The listing builds one solid part. Answer for the finished solid, in the listing's coordinates (mm). Face numbers are marked on the shaded views. Coordinates: 2 decimals unless noted, no trailing zeros. Loops run counter-clockwise (first coordinate to the right, second up) from the corner with the lowest first, then second, coordinate; pieces in that order, holes last. Notation, with made-up numbers: (-19, -29.75) - (5, -29.75) arc R34 cw to (5, 4.25) - close; hole circle Ø3 at (-36, 81). An arc over 180 degrees is marked (long way). Write each question's results on one line, items separated by ' | '. Start each with the question number.
(1) Given pin 1 Ø10.5 at (y, z) = (16, -26) entering from -X; pin 2 Ø5 at (x, z) = (-0.5, 25.4) entering from +Y; pin 3 Ø8 at (y, z) = (23, 2) entering from +X; pin 4 Ø3.5 at (x, z) = (-0.5, -25.4) entering from -Y, each flat-ended and moving along its own axis, determine where each tip first touches the part or whether it passes through.
(2) Find section A-A on y = 21. Determine the outline of the cut face in (x, z), then the cut area to 3 significant figures.
(3) Determine the mould class of the marked faces 1, 2 and 3 for opening direction X: released by +X, released by -X, zero draft, split by the parting line, or undercut.
(4) Find section C-C on z = -6.5. Determine the outline of the cut face in (x, y), then the cut area to 3 significant figures.
(5) Find section D-D on x = -0.5. State how many separate pieces and enclosed holes the cut face has, then the cut area to 3 significant figures.
(6) Consider line 1 (X direction, y = 8, z = 25.4) (3 decimals); line 2 (X direction, y = 6, z = 0) (3 decimals); line 3 (Z direction, x = 13, y = 27). Determine where each line is inside the solid, lowest interval first. Write a range as from..to.
(7) Find section B-B on z = 25.4. Determine the outline of the cut face in (x, y) (3 decimals).
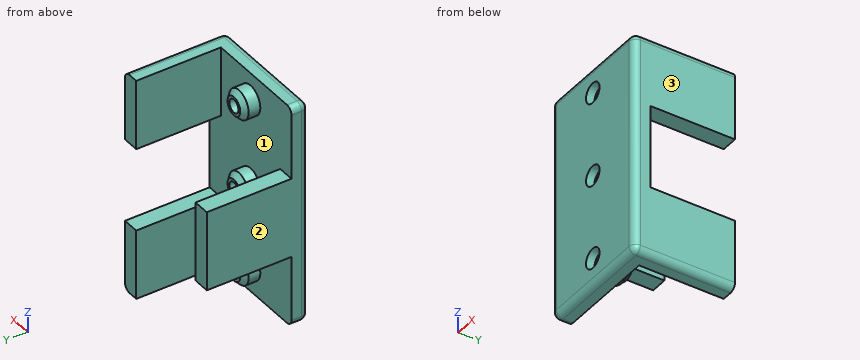
Autodesk Inventor part; units mm, degrees
ref_plane "YZ Plane" through (0, 0, 0) normal (1, 0, 0) x (0, 1, 0)
ref_plane "XZ Plane" through (0, 0, 0) normal (0, 1, 0) x (-1, 0, 0)
ref_plane "XY Plane" through (0, 0, 0) normal (0, 0, 1) x (1, 0, 0)
sketch "Sketch1" plane through (0, 0, 0) normal (0, 1, 0) x (-1, 0, 0)
  line L0 (18.7, 33.5) -> (-17.7, 33.5)
  line L1 (-17.7, 33.5) -> (-17.7, -33.5)
  line L2 (-17.7, -33.5) -> (18.7, -33.5)
  line L3 (18.7, -33.5) -> (18.7, 33.5)
  point P0 (0, 0)
  dimension "d0" = 36.4
  dimension "d1" = 67
extrude "Extrusion1" add sketch "Sketch1" along normal blind 5
sketch "Sketch2" plane through (0, 5, 0) normal (0, 1, 0) x (1, 0, 0)
  line L0 (-18.7, -33.5) -> (17.7, -33.5)
  line L1 (17.7, -33.5) -> (12.7, -33.5)
  line L2 (12.7, -33.5) -> (12.7, -12.5)
  line L3 (12.7, -12.5) -> (17.7, -12.5)
  line L4 (17.7, -12.5) -> (17.7, -33.5)
  line L5 (17.7, -33.5) -> (17.7, 33.5)
  line L6 (17.7, 33.5) -> (12.7, 33.5)
  line L7 (12.7, 33.5) -> (12.7, 12.5)
  line L8 (12.7, 12.5) -> (17.7, 12.5)
  line L9 (17.7, 12.5) -> (17.7, 33.5)
  point P0 (0, 0)
  dimension "d4" = 5
  dimension "d5" = 21
  dimension "d6" = 5
  dimension "d7" = 21
extrude "Extrusion2" add sketch "Sketch2" along normal blind 25.4
fillet "Fillet2" radius 2 6 edges at (-0.5, 0, 33.5) (-18.7, 0, 0) (17.7, 15.2, 33.5) (17.7, 15.2, -33.5) (-0.5, 0, -33.5) (17.7, 0, 0)
sketch "Sketch6" plane through (0, 5, 0) normal (0, 1, 0) x (1, 0, 0)
  line L0 (-18.7, -33.5) -> (-18.7, 33.5)
  line L1 (-18.7, 12) -> (-13.7, 12)
  line L2 (-13.7, 12) -> (-13.7, -12)
  line L3 (-13.7, -12) -> (-18.7, -12)
  line L4 (-18.7, -12) -> (-18.7, 12)
  point P0 (0, 0)
  point P1 (-18.7, -12)
  dimension "d26" = 5
  dimension "d27" = 24
extrude "Extrusion6" add sketch "Sketch6" along normal blind 25.4
fillet "Fillet3" radius 2 4 edges at (-18.1142, 0.5858, 32.9142) (-18.7, 3.5, 33.5) (-18.1142, 0.5858, -32.9142) (-18.7, 3.5, -33.5)
sketch "Sketch8" plane through (0, 5, 0) normal (0, 1, 0) x (1, 0, 0)
  circle A0 centre (-0.5, 0) radius 4.325
  circle A1 centre (-0.5, -25.4) radius 4.325
  circle A2 centre (-0.5, 25.4) radius 4.325
  point P0 (0, 0)
  dimension "d37" = 8.65
  dimension "d38" = 8.65
  dimension "d39" = 8.65
extrude "Extrusion8" add sketch "Sketch8" along normal blind 5
chamfer "Chamfer1" distance 1.5 angle 45 3 edges at (-4.825, 10, 0) (-4.825, 10, -25.4) (-4.825, 10, 25.4)
sketch "Sketch9" plane through (-0.5, 10, 0) normal (0, 1, 0) x (1, 0, 0)
  circle A0 centre (0, 0) radius 2.825
  circle A1 centre (0, 0) radius 2
  circle A2 centre (0, 25.4) radius 2.825
  circle A3 centre (0, 25.4) radius 2
  circle A4 centre (0, -25.4) radius 2.825
  circle A5 centre (0, -25.4) radius 2
  point P0 (0.5, 0)
  dimension "d45" = 4
  dimension "d46" = 4
  dimension "d47" = 4
extrude "Extrusion9" cut sketch "Sketch9" against normal blind 20 contours A1 | A3 | A5
sketch "Sketch10" plane through (0, 0, 0) normal (0, -1, 0) x (1, 0, 0)
  circle A0 centre (-0.5, -25.4) radius 2.825
  circle A1 centre (-0.5, -25.4) radius 3
  circle A2 centre (-0.5, 0) radius 4.325
  circle A3 centre (-0.5, 0) radius 3
  circle A4 centre (-0.5, 25.4) radius 2.825
  circle A5 centre (-0.5, 25.4) radius 3
  point P0 (0, 0)
  dimension "d50" = 6
  dimension "d51" = 6
  dimension "d52" = 6
extrude "Extrusion10" cut sketch "Sketch10" against normal blind 2.5 contours A0 | A1 | A3 | A4 | A5
properties part number "3Wide5mm"
Values:
1) pin 1: stops at x = 12.7 | pin 2: stops at y = 10 | pin 3: stops at x = -13.7 | pin 4: passes through
2) outline: (-18.7, -12) - (-13.7, -12) - (-13.7, 12) - (-18.7, 12) - close; (12.7, -33.5) - (15.7, -33.5) arc R2 ccw to (17.7, -31.5) - (17.7, -12.5) - (12.7, -12.5) - close; (12.7, 12.5) - (17.7, 12.5) - (17.7, 31.5) arc R2 ccw to (15.7, 33.5) - (12.7, 33.5) - close | area: 328 mm²
3) face 1: undercut | face 2: released by -X | face 3: released by +X
4) outline: (-18.7, 2) arc R2 ccw to (-16.7, 0) - (15.7, 0) arc R2 ccw to (17.7, 2) - (17.7, 5) - (-13.7, 5) - (-13.7, 30.4) - (-18.7, 30.4) - close | area: 307 mm²
5) separate pieces: 4 | enclosed holes: 0 | area: 321 mm²
6) line 1: x = -4.825..-2.5, 1.5..3.825, 12.7..17.7 | line 2: x = -18.7..-13.7, -4.825..-2.5, 1.5..3.825 | line 3: z = -33.5..-12.5, 12.5..33.5
7) outline: (-18.7, 2) arc R2 ccw to (-16.7, 0) - (-3.5, 0) - (-3.5, 2.5) - (-2.5, 2.5) - (-2.5, 10) - (-3.325, 10) - (-4.825, 8.5) - (-4.825, 5) - (-18.7, 5) - close; (1.5, 2.5) - (2.5, 2.5) - (2.5, 0) - (15.7, 0) arc R2 ccw to (17.7, 2) - (17.7, 30.4) - (12.7, 30.4) - (12.7, 5) - (3.825, 5) - (3.825, 8.5) - (2.325, 10) - (1.5, 10) - close
